Source: CAD feature listing. Evaluate the final solid. Frame: model axes, mm. Face numbers are marked on the shaded views. A direction names the side the tool comes from. Round coordinates to 2 decimals unless told otherwise and drop trailing zeros. Order: outer loops, then holes, each group sorted by start corner. A loop starts at its lowest first (then second) coordinate and runs counter-clockwise, first axis right, second up. Notation, with made-up numbers: M -11,73 L 1,73 A22 ccw 1,109 Z; hole C 85,66 d7. An arc over 180 degrees is marked long. Answer in a Markdown table with one row per item. Add a question column.
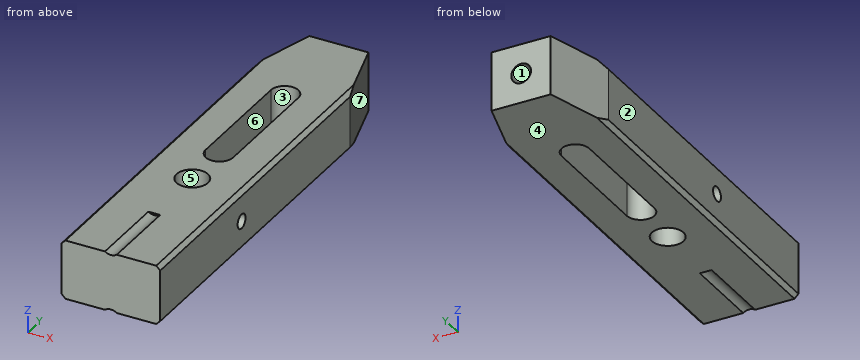
```python
from build123d import *

# Parameters (mm, degrees)
SKETCH2_W           = 50
SKETCH2_H           = 30
BOSS_EXTRUDE2_DEPTH = 210
CUT_EXTRUDE2_REACH  = 32
SKETCH3_R           = 8
CUT_EXTRUDE5_REACH  = 32
CUT_EXTRUDE8_REACH  = 32
CHAMFER3_SIZE       = 2
CUT_EXTRUDE10_DEPTH = 40
SKETCH16_R          = 3.65
CUT_EXTRUDE11_DEPTH = 50
SKETCH20_R          = 5
CUT_EXTRUDE13_DEPTH = 35


with BuildPart() as part:
    # Sketch2 → Boss-Extrude2 (new body)
    with BuildSketch(Plane(origin=(0, 0, 0), x_dir=(1, 0, 0), z_dir=(0, 1, 0))):
        with Locations((25, 15)):
            Rectangle(SKETCH2_W, SKETCH2_H)
    extrude(amount=BOSS_EXTRUDE2_DEPTH)

    # Sketch3 → Cut-Extrude2 (cut, up to next)
    with BuildSketch(Plane.XY, mode=Mode.PRIVATE) as cut_extrude2_sk1:
        with Locations((25, 75)):
            Circle(SKETCH3_R)
    cut_extrude2_tool1 = extrude(cut_extrude2_sk1.sketch, amount=-CUT_EXTRUDE2_REACH, mode=Mode.PRIVATE) & part.part
    add(cut_extrude2_tool1.solids().sort_by_distance((25, 75, 0))[0], mode=Mode.SUBTRACT)

    # Sketch7 → Cut-Extrude5 (cut, up to next)
    with BuildSketch(Plane.XY, mode=Mode.PRIVATE) as cut_extrude5_sk1:
        Polygon((0, 175), (10, 210), (0, 210), align=None)
    cut_extrude5_tool1 = extrude(cut_extrude5_sk1.sketch, amount=-CUT_EXTRUDE5_REACH, mode=Mode.PRIVATE) & part.part
    add(cut_extrude5_tool1.solids().sort_by_distance((3.333333, 198.333333, 0))[0], mode=Mode.SUBTRACT)
    # Sketch7 → Cut-Extrude5 (cut, up to next)
    with BuildSketch(Plane.XY, mode=Mode.PRIVATE) as cut_extrude5_sk2:
        Polygon((50, 210), (50, 175), (40, 210), align=None)
    cut_extrude5_tool2 = extrude(cut_extrude5_sk2.sketch, amount=-CUT_EXTRUDE5_REACH, mode=Mode.PRIVATE) & part.part
    add(cut_extrude5_tool2.solids().sort_by_distance((46.666667, 198.333333, 0))[0], mode=Mode.SUBTRACT)

    # Sketch11 → Cut-Extrude8 (cut, up to next)
    with BuildSketch(Plane(origin=(0, 0, -30), x_dir=(-1, 0, 0), z_dir=(0, 0, -1)), mode=Mode.PRIVATE) as cut_extrude8_sk1:
        with BuildLine():
            Line((-18, 160), (-18, 100))
            ThreePointArc((-18, 100), (-25, 93), (-32, 100))
            Line((-32, 100), (-32, 160))
            ThreePointArc((-32, 160), (-25, 167), (-18, 160))
        make_face()
    cut_extrude8_tool1 = extrude(cut_extrude8_sk1.sketch, amount=-CUT_EXTRUDE8_REACH, mode=Mode.PRIVATE) & part.part
    add(cut_extrude8_tool1.solids().sort_by_distance((25, 130, -30))[0], mode=Mode.SUBTRACT)

    # Chamfer3
    chamfer3_edges = [part.edges().sort_by_distance(p)[0] for p in [
        (0, 87.5, -30),
        (50, 87.5, -30),
        (50, 87.5, 0),
        (0, 87.5, 0),
    ]]
    chamfer(chamfer3_edges, length=CHAMFER3_SIZE)

    # Sketch15 → Cut-Extrude10 (cut)
    with BuildSketch(Plane.XZ):
        with BuildLine():
            Line((22, 0), (28, 0))
            ThreePointArc((28, 0), (25, -1), (22, 0))
        make_face()
        with BuildLine():
            Line((22, -30), (28, -30))
            ThreePointArc((28, -30), (25, -29), (22, -30))
        make_face()
    extrude(amount=-CUT_EXTRUDE10_DEPTH, mode=Mode.SUBTRACT)

    # Sketch16 → Cut-Extrude11 (cut)
    with BuildSketch(Plane(origin=(50, 0, 0), x_dir=(0, 0, -1), z_dir=(1, 0, 0))):
        with Locations((15, 75)):
            Circle(SKETCH16_R)
    extrude(amount=-CUT_EXTRUDE11_DEPTH, mode=Mode.SUBTRACT)

    # Sketch20 → Cut-Extrude13 (cut)
    with BuildSketch(Plane(origin=(0, 210, 0), x_dir=(1, 0, 0), z_dir=(0, 1, 0))):
        with Locations((25, 15)):
            Circle(SKETCH20_R)
    extrude(amount=-CUT_EXTRUDE13_DEPTH, mode=Mode.SUBTRACT)


solid = part.part
```
(1) Line query: line 1 (Y direction, x = 25, z = -7); line 2 (Y direction, x = 25, z = -17); line 3 (X direction, y = 139.5, z = -24.5). Output: solid intervals per line, ascending. Write a range as from..to.
(2) Access query for the marked faces 1, 2 and 3. Directions: +Z, -Z, +X, -X, +Y, -Y. A direction counts if a zero-diameter tool reaches every point of the face in a straight line with its end or side. Return the directions, or none.
(3) Cut plane C-C (y = 144.5). Return loops of the section in (x, z).
(4) Cut plane B-B (x = 25). Return loops of the section in (y, z), and give its area (3 significant figures).
(5) Pin query (flat end, axial travel): pin 1 (6 mm diameter, centred on y = 188.5, z = -15.5, fed in from -X). Return the tip coordinate at first contact, or that it passes through.
(6) Cut plane D-D (z = -24). Return loops of the section in (x, y), and give its area (4 significant figures).
(7) Cut plane A-A (z = -15). Return loops of the section in (x, y).
(8) Draft query along Y for the marked faces 4, 5, 6 and 7. Return one class per face: +Y half, -Y half, draft (parallel to the pull), parting line (faces both ways), or undercut.
Answer list:
| question | item | result |
|---|---|---|
| 1 | line 1 | 0..67, 83..93, 167..210 |
| 1 | line 2 | 0..67, 83..93, 167..175 |
| 1 | line 3 | 0..18, 32..50 |
| 2 | face 1 | +Y |
| 2 | face 2 | +Z, -Z, -X, +Y, -Y |
| 2 | face 3 | +Z, -Z |
| 3 | outline | M 0,-28 L 2,-30 L 18,-30 L 18,0 L 2,0 L 0,-2 Z; M 32,-30 L 48,-30 L 50,-28 L 50,-2 L 48,0 L 32,0 Z |
| 4 | outline | M 0,-29 L 40,-29 L 40,-30 L 67,-30 L 67,0 L 40,0 L 40,-1 L 0,-1 Z; M 83,-30 L 93,-30 L 93,0 L 83,0 Z; M 167,-30 L 210,-30 L 210,-20 L 175,-20 L 175,-10 L 210,-10 L 210,0 L 167,0 Z |
| 4 | area | 3,170 mm² |
| 5 | pin 1 | x = 3 |
| 6 | outline | M 0,0 L 50,0 L 50,175 L 40,210 L 10,210 L 0,175 Z; hole C 25,75 d16; hole M 18,100 A7 ccw 32,100 L 32,160 A7 ccw 18,160 Z |
| 6 | area | 8,955 mm² |
| 7 | outline | M 0,0 L 50,0 L 50,71.35 L 32.12,71.35 A8 cw 17.88,71.35 L 0,71.35 Z; M 0,78.65 L 17.88,78.65 A8 cw 32.12,78.65 L 50,78.65 L 50,175 L 40,210 L 30,210 L 30,175 L 20,175 L 20,210 L 10,210 L 0,175 Z; hole M 18,100 A7 ccw 32,100 L 32,160 A7 ccw 18,160 Z |
| 8 | face 4 | draft |
| 8 | face 5 | undercut |
| 8 | face 6 | undercut |
| 8 | face 7 | +Y half |
